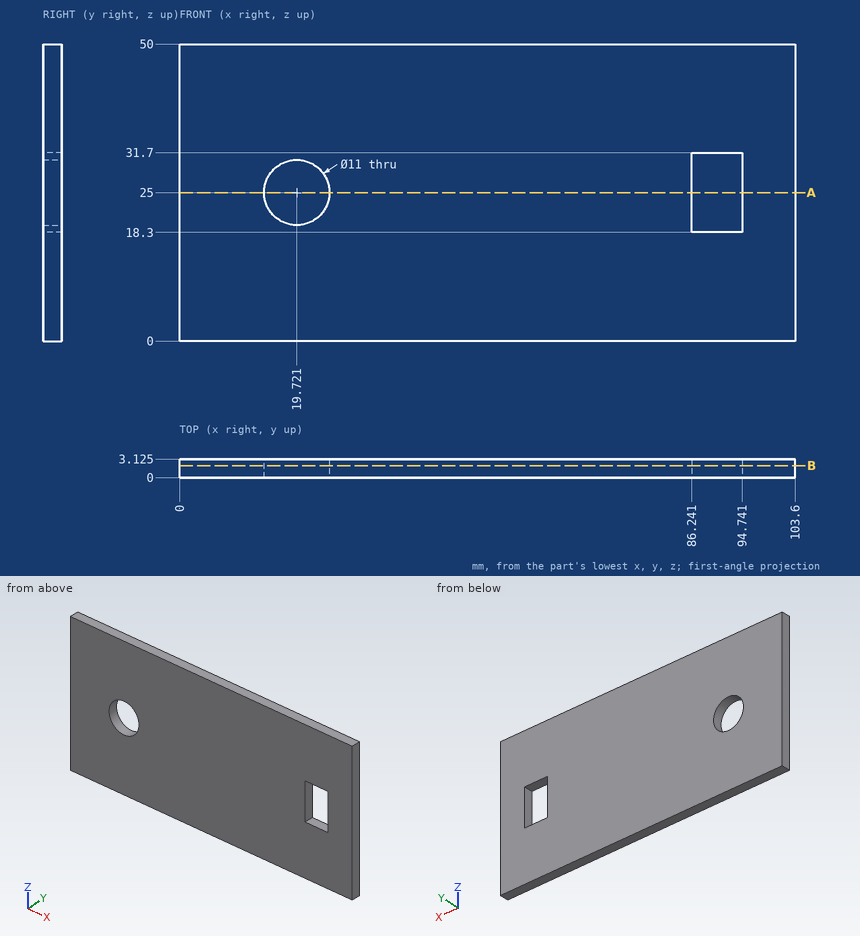
Part print with two shaded views. Sizes in mm from the minimum x, y, z corner. Give positions to 0.01 mm unless a question says otherwise; leave off trailing zeros. Loops run counter-clockwise (first coordinate to the right, second up) from the corner with the lowest first, then second, coordinate; pieces in that order, holes last. Notation, with made-up numbers: (64, 9.5) - (77, 9.5) arc R25 cw to (77, 46.5) - close; hole circle Ø6 at (80.5, -22). An arc over 180 degrees is marked (long way). Put each result on its own line as item: value.
Q1. Slice it at A-A (z = 25). Give the cut face in (x, y) (1 decimal).
Filled in:
outline: (0, 0) - (14.2, 0) - (14.2, 3.1) - (0, 3.1) - close; (25.2, 0) - (86.2, 0) - (86.2, 3.1) - (25.2, 3.1) - close; (94.7, 0) - (103.6, 0) - (103.6, 3.1) - (94.7, 3.1) - close
Q2. Probe line 1 along X through (y, z) = (1.1, 25); line 2 along X through (y, z) = (0.7, 19); line 3 along X through (y, z) = (1.9, 24). List the from-to ranges inside material, lowest first.
Filled in:
line 1: x = 0 to 14.22, 25.22 to 86.24, 94.74 to 103.6
line 2: x = 0 to 86.24, 94.74 to 103.6
line 3: x = 0 to 14.31, 25.13 to 86.24, 94.74 to 103.6
Q3. Slice it at B-B (y = 2). Give the cut face in (x, z), plus the area to 3 significant figures.
Filled in:
outline: (0, 0) - (103.6, 0) - (103.6, 50) - (0, 50) - close; hole circle Ø11 at (19.72, 25); hole (86.24, 18.3) - (94.74, 18.3) - (94.74, 31.7) - (86.24, 31.7) - close
area: 4,970 mm²
